Geometry check sheet. Reference: the model listing, model coordinates, mm. Round coordinates to 2 decimals unless told otherwise and drop trailing zeros. Loops run counter-clockwise (first coordinate to the right, second up) from the corner with the lowest first, then second, coordinate; pieces in that order, holes last. Notation, with made-up numbers: (80.5, 6.25) - (95.5, 6.25) arc R30 ccw to (95.5, 39.25) - close; hole circle Ø1 at (59.5, 83.25). An arc over 180 degrees is marked (long way). Answer as CSV lines item,"result". Start each with the question number.
1) Cross-section at B-B on y = 10. Record the boundary of the cut face in (x, z), and give its area (3 significant figures).
2) Depth check by flat-ended pin: P1, Ø10.5, axis at y = 10, z = 30, coming from the -X side; P2, Ø5, axis at y = 3.5, z = -4.5, coming from the +X side; P3, Ø5, axis at y = 10, z = -30, coming from the +X side. Enter the tip coordinate at first touch or a pass-through.
3) Cross-section at A-A on z = 30. Record the boundary of the cut face in (x, y).
4) Draft check along Y on faces 1 (the cylindrical face through (-15.496, 9.86, 0.341)), 2 (the flat face through (-16, 0, 1)), 3 (the flat face through (-16, 20, 1)), 4 (the cylindrical face through (-9.89, 11.22, 33.86)). Enter one of: released by +Y, released by -Y, zero draft, split by the parting line, or undercut.
5) Cross-section at D-D on x = -9. Record the boundary of the cut face in (y, z).
6) Cross-section at C-C on x = -12. Record the boundary of the cut face in (y, z).
7) Thickness scan on line 1 along Y through (x, z) = (-5.5, -30); line 2 along Z through (x, y) = (-1.25, 8.25); line 3 along Z through (x, y) = (-6.75, 13.5). Record the ranges inside material, lowest first.
Autodesk Inventor part; units mm, degrees
ref_plane "YZ Plane" through (0, 0, 0) normal (1, 0, 0) x (0, 1, 0)
ref_plane "XZ Plane" through (0, 0, 0) normal (0, 1, 0) x (-1, 0, 0)
ref_plane "XY Plane" through (0, 0, 0) normal (0, 0, 1) x (1, 0, 0)
sketch "Sketch3" plane through (0, 0, 0) normal (0, 1, 0) x (-1, 0, 0)
  arc A0 (0, -15.5) -> (0, 15.5) centre (0, 0) ccw
  line L0 (0, 15.5) -> (0, 36)
  line L1 (0, -15.5) -> (0, -36)
  line L2 (0, 36) -> (19.5, 36)
  line L3 (19.5, 36) -> (19.5, -36)
  line L4 (19.5, -36) -> (0, -36)
  dimension "d17" = 31
  dimension "d19" = 20.5
  dimension "d20" = 20.5
extrude "Extrusion3" add sketch "Sketch3" along normal blind 20
ref_plane "Work Plane2" through (-19.5, 0, -36) normal (-1, 0, 0) x (0, 0, 1)
sketch "Sketch4" plane through (-19.5, 0, -36) normal (-1, 0, 0) x (0, 0, 1)
  line L0 (0, 0) -> (0, 20)
  line L1 (0, 10) -> (6, 10)
  line L2 (72, 0) -> (72, 20)
  line L3 (72, 10) -> (66, 10)
  circle A0 centre (6, 10) radius 4.05
  circle A1 centre (66, 10) radius 4.05
  point P0 (36, 0)
  dimension "d25" = 6
  dimension "d26" = 6
  dimension "d27" = 8.1
  dimension "d28" = 8.1
extrude "Extrusion4" cut sketch "Sketch4" against normal blind 20
properties part number "mounpt2"
Answer block:
1,outline,"(-19.5, -36) - (0, -36) - (0, -34.05) - (-19.5, -34.05) - close; (-19.5, -25.95) - (0, -25.95) - (0, -15.5) arc R15.5 cw to (0, 15.5) - (0, 25.95) - (-19.5, 25.95) - close; (-19.5, 34.05) - (0, 34.05) - (0, 36) - (-19.5, 36) - close"
1,area,"711 mm^2"
2,P1,"stops at x = -19.5"
2,P2,"stops at x = -13.83"
2,P3,"passes through"
3,outline,"(-19.5, 0) - (0, 0) - (0, 5.95) - (-19.5, 5.95) - close; (-19.5, 14.05) - (0, 14.05) - (0, 20) - (-19.5, 20) - close"
4,face 1,"zero draft"
4,face 2,"released by -Y"
4,face 3,"released by +Y"
4,face 4,"undercut"
5,outline,"(0, -36) - (20, -36) - (20, -12.62) - (0, -12.62) - close; (0, 12.62) - (20, 12.62) - (20, 36) - (0, 36) - close; hole circle Ø8.1 at (10, -30); hole circle Ø8.1 at (10, 30)"
6,outline,"(0, -36) - (20, -36) - (20, -9.81) - (0, -9.81) - close; (0, 9.81) - (20, 9.81) - (20, 36) - (0, 36) - close; hole circle Ø8.1 at (10, -30); hole circle Ø8.1 at (10, 30)"
7,line 1,"y = 0 to 5.95, 14.05 to 20"
7,line 2,"z = -36 to -33.65, -26.35 to -15.45, 15.45 to 26.35, 33.65 to 36"
7,line 3,"z = -36 to -32.04, -27.96 to -13.95, 13.95 to 27.96, 32.04 to 36"
